from build123d import *

# Parameters (mm, degrees)
F0_R            = 31.75
F0_R_2          = 14.1605
F1_DEPTH        = 3.175
F2_R            = 2.3622
F3_DEPTH        = 3.176
F3_COPIES_COUNT = 6


# Not quite as in the source:
# - a pattern or mirror of a feature is missing from the dataset's text; its kind, count and spacing are read off the source's solid


with BuildPart() as f1:
    # F0 (on Top) → F1 (new body)
    with BuildSketch(Plane.XY):
        Circle(F0_R)
        Circle(F0_R_2, mode=Mode.SUBTRACT)
    extrude(amount=F1_DEPTH)

    # F2 (on face) → F3 (cut, through all)
    with BuildSketch(Plane.XY.offset(3.175)):
        with Locations((0, 23.8125)):
            Circle(F2_R)
    f3 = extrude(amount=-F3_DEPTH, mode=Mode.SUBTRACT)

    # F3_copies: F3 ×6 about axis
    f3_copies_axis = Axis((0, 0, 0), (0, 0, 1))
    for i in range(1, F3_COPIES_COUNT):
        add(f3.rotate(f3_copies_axis, i * 360 / F3_COPIES_COUNT), mode=Mode.SUBTRACT)


solid = f1.part
Can you work these out from the model? Positions are in its coordinate system, mm. Round coordinates to 2 decimals unless told otherwise and drop trailing zeros. Order: outer loops, then holes, each group sorted by start corner. A loop starts at its lowest first (then second) coordinate and runs counter-clockwise, first axis right, second up. Notation, with made-up numbers: M -1.75,71 L 55.25,71 A25 cw 55.25,87 Z; hole C 17.25,21 d3. An arc over 180 degrees is marked long. Use a Markdown table: item, result.
1) Imagine slicing it at D-D (y = -6.5). List the corners of the cut face in (x, z) for me (3 decimals).
Geometry says:
| item | result |
|---|---|
| outline | M -31.078,0 L -12.581,0 L -12.581,3.175 L -31.078,3.175 Z; M 12.581,0 L 31.078,0 L 31.078,3.175 L 12.581,3.175 Z |
2) If I drill on line 1 along Y through (x, z) = (0, 1); line 2 along Y through (x, z) = (-2, 2.45); line 3 along X through (y, z) = (-13, 1.65), over which ranges is the centre line in solid material (lowest first)?
Geometry says:
| item | result |
|---|---|
| line 1 | y = -31.75 to -26.17, -21.45 to -14.16, 14.16 to 21.45, 26.17 to 31.75 |
| line 2 | y = -31.69 to -25.07, -22.56 to -14.02, 14.02 to 22.56, 25.07 to 31.69 |
| line 3 | x = -28.97 to -22.72, -18.53 to -5.61, 5.61 to 18.53, 22.72 to 28.97 |
3) If we mould it in two halves opening along Y, with no side actions, what happens to faces 1 (the face through (14, -7, 3.175)), 2 (the face through (22.875, -11.197, 1.61)), 3 (the face through (-6.883, -30.995, 1.565))? For each: +Y half, -Y half, draft (parallel to the pull), parting line (faces both ways), or undercut.
Geometry says:
| item | result |
|---|---|
| face 1 | draft |
| face 2 | undercut |
| face 3 | parting line |
4) Imagine slicing it at C-C (z = 1.7). List the corners of the cut face in (x, y) for me, then the cut area to 3 significant figures.
Geometry says:
| item | result |
|---|---|
| outline | C 0,0 d63.5; hole C -20.62,-11.91 d4.72; hole C -20.62,11.91 d4.72; hole C 0,0 d28.32; hole C 0,-23.81 d4.72; hole C 0,23.81 d4.72; hole C 20.62,-11.91 d4.72; hole C 20.62,11.91 d4.72 |
| area | 2,430 mm² |
5) I'm going to push flat-ended pins straight in: P1, Ø2, axis at x = -18, y = -22, coming from the -Z side; P2, Ø4, axis at x = -20.62, y = 11.91, coming from the +Z side; P3, Ø1.5, axis at y = 9, z = 1, coming from the -X side. Where does each tip first touch, or does it pass through?
Geometry says:
| item | result |
|---|---|
| P1 | stops at z = 0 |
| P2 | passes through |
| P3 | stops at x = -30.66 |
6) Imagine slicing it at B-B (x = 0). Give the number of separate pieces and of enclosed holes in the cut face, then the cut area to 3 significant figures.
Geometry says:
| item | result |
|---|---|
| separate pieces | 4 |
| enclosed holes | 0 |
| area | 81.7 mm² |
